```python
from build123d import *

# Parameters (mm, degrees)
EXTRUDE_1_DEPTH           = 270
HOLE_WIZARD_1_D           = 4.5
HOLE_WIZARD_1_CBORE_D     = 8
HOLE_WIZARD_1_CBORE_DEPTH = 4.5
PATTERN_LINEAR_1_COUNT    = 7
PATTERN_LINEAR_1_PITCH    = 40


with BuildPart() as part:
    # 草图1 → 凸台-拉伸1 (new body)
    with BuildSketch(Plane.XY):
        with BuildLine():
            Line((-12, 3), (-12, 3.85))
            Line((-12, 3.85), (-11.6, 4.25))
            Line((-11.6, 4.25), (11.6, 4.25))
            Line((11.6, 4.25), (12, 3.85))
            Line((12, 3.85), (12, 3))
            ThreePointArc((12, 3), (10.75, 1.75), (12, 0.5))
            Line((12, 0.5), (12, -3.85))
            Line((12, -3.85), (11.6, -4.25))
            Line((11.6, -4.25), (6.3, -4.25))
            ThreePointArc((6.3, -4.25), (6, -3.95), (5.7, -4.25))
            Line((5.7, -4.25), (-11.6, -4.25))
            Line((-11.6, -4.25), (-12, -3.85))
            Line((-12, -3.85), (-12, 0.5))
            ThreePointArc((-12, 0.5), (-10.75, 1.75), (-12, 3))
        make_face()
    extrude(amount=-EXTRUDE_1_DEPTH)

    # 打孔尺寸根据内六角圆柱头螺钉的类型1 (through all)
    with Locations(Plane(origin=(0, 4.25, 0), x_dir=(1, 0, 0), z_dir=(0, 1, 0))):
        with Locations((0, 15)):
            hole_wizard_1 = CounterBoreHole(HOLE_WIZARD_1_D / 2, HOLE_WIZARD_1_CBORE_D / 2, HOLE_WIZARD_1_CBORE_DEPTH)

    # 阵列(线性)1: 打孔尺寸根据内六角圆柱头螺钉的类型1 ×7
    with Locations(*[(0, 0, -i * PATTERN_LINEAR_1_PITCH) for i in range(1, PATTERN_LINEAR_1_COUNT)]):
        add(hole_wizard_1, mode=Mode.SUBTRACT)


solid = part.part
```
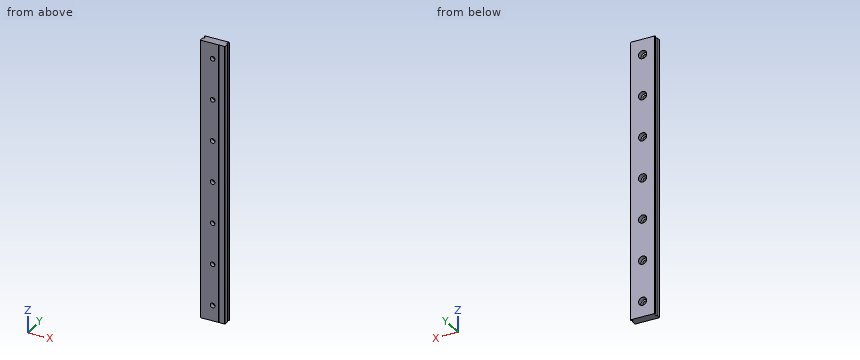
Build history of the part. All positions in model axes, mm. Round coordinates to 2 decimals unless told otherwise and drop trailing zeros. Write each loop counter-clockwise with the first axis right and the second up, starting at its lowest first coordinate (ties: lowest second). Pieces come first, ordered by that corner, then holes. Notation, with made-up numbers: (87, 25) -> (139, 25) arc R29 ccw to (139, 64) -> close; hole circle Ø5 at (-27.75, 20). An arc over 180 degrees is marked (long way). Put each result on its own line as item: value.
Item 1: Slice it at D-D, the plane x = 0. Count the separate pieces of the cut face and the enclosed holes in it, plus the area to 3 significant figures.
Here are the results:
separate pieces: 8
enclosed holes: 0
area: 1,920 mm^2
Item 2: Slice it at A-A, the plane z = -55. Give the cut face in (x, y).
Here are the results:
outline: (-12, -3.85) -> (-11.6, -4.25) -> (-2.25, -4.25) -> (-2.25, -0.25) -> (-4, -0.25) -> (-4, 4.25) -> (-11.6, 4.25) -> (-12, 3.85) -> (-12, 3) arc R1.25 cw to (-12, 0.5) -> close; (2.25, -4.25) -> (5.7, -4.25) arc R0.3 cw to (6.3, -4.25) -> (11.6, -4.25) -> (12, -3.85) -> (12, 0.5) arc R1.25 cw to (12, 3) -> (12, 3.85) -> (11.6, 4.25) -> (4, 4.25) -> (4, -0.25) -> (2.25, -0.25) -> close
Item 3: Flat gauge pin, fed straight in: P1, Ø6.5, axis at x = 0, z = -55, coming from the +Y side. Where does the tip first touch, or does it go through?
Here are the results:
P1: stops at y = -0.25
Item 4: Slice it at C-C, the plane z = -142. Give the cut face in (x, y), plus the area to 3 significant figures.
Here are the results:
outline: (-12, -3.85) -> (-11.6, -4.25) -> (5.7, -4.25) arc R0.3 cw to (6.3, -4.25) -> (11.6, -4.25) -> (12, -3.85) -> (12, 0.5) arc R1.25 cw to (12, 3) -> (12, 3.85) -> (11.6, 4.25) -> (-11.6, 4.25) -> (-12, 3.85) -> (-12, 3) arc R1.25 cw to (-12, 0.5) -> close
area: 199 mm^2
Item 5: Slice it at B-B, the plane y = -2.5. Give the cut face in (x, z).
Here are the results:
outline: (-12, -270) -> (12, -270) -> (12, 0) -> (-12, 0) -> close; hole circle Ø4.5 at (0, -255); hole circle Ø4.5 at (0, -215); hole circle Ø4.5 at (0, -175); hole circle Ø4.5 at (0, -135); hole circle Ø4.5 at (0, -95); hole circle Ø4.5 at (0, -55); hole circle Ø4.5 at (0, -15)
Item 6: Wall check: probe 1 along X at (y, z) = (1.8, -255); probe 2 along X at (y, z) = (-2.3, -215); probe 3 along Y at (x, z) = (11.25, -185.5). Give the ranges that are in metal, low to high. Write a range as from..to.
Here are the results:
probe 1: x = -10.75..-4, 4..10.75
probe 2: x = -12..-2.25, 2.25..12
probe 3: y = -4.25..0.75, 2.75..4.25
